Can you work these out from the drawing? Everything is in mm from the part's minimum corner. A direction names the side the tool comes from. Coordinates: 2 decimals unless noted, no trailing zeros. Loops run counter-clockwise (first coordinate to the right, second up) from the corner with the lowest first, then second, coordinate; pieces in that order, holes last. Notation, with made-up numbers: (45, -34.75) -> (54, -34.75) arc R29 ccw to (54, 4.25) -> close; hole circle Ø8 at (78.25, 14). An arc over 180 degrees is marked (long way). Put each result on its own line as item: value. Start each with the question number.
Item 1: Will these pins go through, and if not, where does the flat tip stop? P1, Ø3, axis at y = 10.5, z = 2, coming from the -X side; P2, Ø1, axis at x = 33.5, y = 10, coming from the +Z side; P3, Ø5, axis at x = 81, z = 4, coming from the -Y side; P4, Ø5, axis at x = 65, z = 5.5, coming from the +Y side.
Item 2: If we section it at A-A on y = 12: Please give me the cut outline in (x, z), plus the area to 3 significant figures.
Item 3: If we section it at C-C on y = 1.5: Please give me the cut outline in (x, z), plus the area to 3 significant figures.
Item 4: If we section it at B-B on x = 112: Please give me the cut outline in (y, z), plus the area to 3 significant figures.
Item 5: For the marked faces 3 and 4, which set-ups out of +Z, -Z, +X, -X, +Y, -Y let a thin tool reach every point of the face, with its end or its side?
Item 6: We'd pull the mould along X, two halves only. Please class the marked faces 1 and 2: pulls with the +X half, pulls with the -X half, needs draft (parallel to the pull), parting line crosses it, or undercut.
Item 7: If we section it at D-D on x = 72.5: Please give me the cut outline in (y, z).
Item 8: Please list where these lines run through material, in increasing order: L1, parallel to Y at x = 12, z = 2.7; L2, parallel to X at y = 15, z = 3; L3, parallel to Z at x = 88.5, y = 10.75. Write a range as from..to.
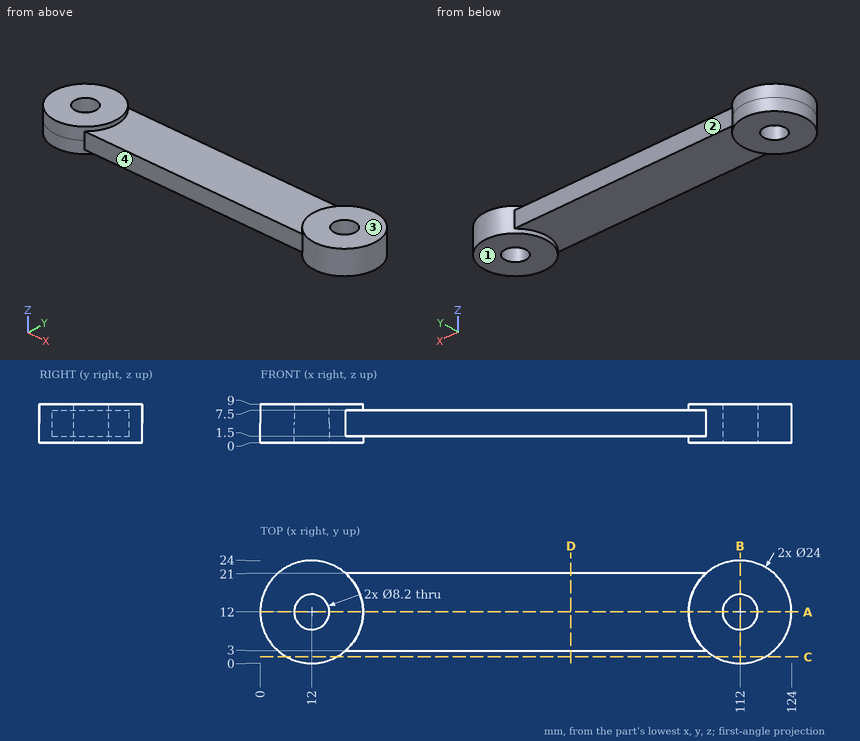
Solutions:
1. P1: x = 0
1. P2: z = 7.5
1. P3: y = 3
1. P4: y = 21
2. outline: (0, 0) -> (7.9, 0) -> (7.9, 9) -> (0, 9) -> close; (16.1, 0) -> (24, 0) -> (24, 1.5) -> (100, 1.5) -> (100, 0) -> (107.9, 0) -> (107.9, 9) -> (100, 9) -> (100, 7.5) -> (24, 7.5) -> (24, 9) -> (16.1, 9) -> close; (116.1, 0) -> (124, 0) -> (124, 9) -> (116.1, 9) -> close
2. area: 740 mm^2
3. outline: (6.19, 0) -> (17.81, 0) -> (17.81, 9) -> (6.19, 9) -> close; (106.19, 0) -> (117.81, 0) -> (117.81, 9) -> (106.19, 9) -> close
3. area: 209 mm^2
4. outline: (0, 0) -> (7.9, 0) -> (7.9, 9) -> (0, 9) -> close; (16.1, 0) -> (24, 0) -> (24, 9) -> (16.1, 9) -> close
4. area: 142 mm^2
5. face 3: +Z, +X, -X, +Y, -Y
5. face 4: +Z, -Z, -Y
6. face 1: needs draft
6. face 2: undercut
7. outline: (3, 1.5) -> (21, 1.5) -> (21, 7.5) -> (3, 7.5) -> close
8. L1: 0..7.9, 16.1..24
8. L2: 0.38..9.21, 14.79..109.21, 114.79..123.62
8. L3: 1.5..7.5
